```python
from build123d import *

# Parameters (mm, degrees)
F0_R     = 19.05
F0_R_2   = 6.35
F1_DEPTH = 134.62
F0_R_3   = 31.75
F2_DEPTH = 65.024
F3_R     = 5.08
F4_DEPTH = 114.3
F5_DEPTH = 89.662


with BuildPart() as f1:
    # F0 (on Front) → F1 (new body)
    with BuildSketch(Plane.XZ):
        Circle(F0_R)
        Circle(F0_R_2, mode=Mode.SUBTRACT)
    extrude(amount=F1_DEPTH)

    # F0 (on Front) → F2 (join)
    with BuildSketch(Plane.XZ):
        Circle(F0_R_3)
        Circle(F0_R, mode=Mode.SUBTRACT)
    extrude(amount=F2_DEPTH)

    # F3 (on Right) → F4 (cut)
    with BuildSketch(Plane.YZ):
        with Locations((-15.709256, 0)):
            Circle(F3_R)
        with Locations((-36.759584, 0)):
            Circle(F3_R)
    extrude(amount=-F4_DEPTH, mode=Mode.SUBTRACT)

    # F3 (on Right) → F5 (cut)
    with BuildSketch(Plane.YZ):
        with Locations((-15.709256, 0)):
            Circle(F3_R)
        with Locations((-36.759584, 0)):
            Circle(F3_R)
    extrude(amount=F5_DEPTH, mode=Mode.SUBTRACT)


solid = f1.part
```
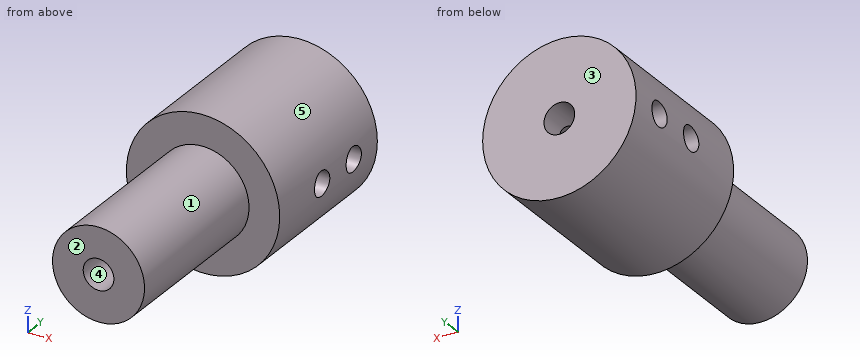
Can you work these out from the model? Positions are in its coordinate system, mm. Face numbers are marked on the shaded views. A direction names the side the tool comes from. Coordinates: 2 decimals unless noted, no trailing zeros. Order: outer loops, then holes, each group sorted by start corner. A loop starts at its lowest first (then second) coordinate and runs counter-clockwise, first axis right, second up. Notation, with made-up numbers: (-0.75, 35.25) -> (26.25, 35.25) arc R19 ccw to (26.25, 53.25) -> close; hole circle Ø5 at (56, -0.75). An arc over 180 degrees is marked (long way). Write each question's results on one line, items separated by ' | '.
Item 1: I want a section at B-B, the plane z = 0. Write out the boundary of the cut face in (x, y).
Results are:
outline: (-31.75, -65.02) -> (-19.05, -65.02) -> (-19.05, -134.62) -> (-6.35, -134.62) -> (-6.35, -41.84) -> (-31.75, -41.84) -> close; (-31.75, -31.68) -> (-6.35, -31.68) -> (-6.35, -20.79) -> (-31.75, -20.79) -> close; (-31.75, -10.63) -> (-6.35, -10.63) -> (-6.35, 0) -> (-31.75, 0) -> close; (6.35, -134.62) -> (19.05, -134.62) -> (19.05, -65.02) -> (31.75, -65.02) -> (31.75, -41.84) -> (6.35, -41.84) -> close; (6.35, -31.68) -> (31.75, -31.68) -> (31.75, -20.79) -> (6.35, -20.79) -> close; (6.35, -10.63) -> (31.75, -10.63) -> (31.75, 0) -> (6.35, 0) -> close
Item 2: I want a section at D-D, the plane x = 9.5. Write out the boundary of the cut face in (y, z).
Results are:
outline: (-134.62, -16.51) -> (-65.02, -16.51) -> (-65.02, -30.3) -> (0, -30.3) -> (0, 30.3) -> (-65.02, 30.3) -> (-65.02, 16.51) -> (-134.62, 16.51) -> close; hole circle Ø10.16 at (-36.76, 0); hole circle Ø10.16 at (-15.71, 0)
Item 3: I'm going to push flat-ended pins straight in: pin 1 Ø6 at (y, z) = (-91.5, 7) entering from -X; pin 2 Ø16.5 at (y, z) = (-15.71, 0) entering from +X; pin 3 Ø1 at (y, z) = (-98, -13.5) entering from +X; pin 4 Ø5 at (y, z) = (-63.5, -24) entering from +X. Where does each tip first touch, or does it pass through?
Results are:
pin 1: x = -18.63 | pin 2: x = 31.75 | pin 3: x = 13.92 | pin 4: x = 23.36
Item 4: I want a section at C-C, the plane y = -89. Write out the boundary of the cut face in (x, z), then the cut area to 3 significant figures.
Results are:
outline: circle Ø38.1 at (0, 0); hole circle Ø12.7 at (0, 0) | area: 1,010 mm²
Item 5: If we mould it in two halves opening along Z, with no side actions, what happens to the marked faces 3, 4 and 5? For each: +Z half, -Z half, draft (parallel to the pull), parting line (faces both ways), or undercut.
Results are:
face 3: draft | face 4: undercut | face 5: parting line
Item 6: If I drill on line 1 along Y through (x, z) = (20, 0); line 2 along Z through (x, y) = (0, -97); line 3 along Z through (x, y) = (0.5, -9), over which ranges is the centre line in solid material (lowest first)?
Results are:
line 1: -65.02 to -41.84, -31.68 to -20.79, -10.63 to 0 | line 2: -19.05 to -6.35, 6.35 to 19.05 | line 3: -31.75 to -6.33, 6.33 to 31.75
Item 7: I want a section at A-A, the plane x = 0. Write out the boundary of the cut face in (y, z).
Results are:
outline: (-134.62, -19.05) -> (-65.02, -19.05) -> (-65.02, -31.75) -> (0, -31.75) -> (0, -6.35) -> (-134.62, -6.35) -> close; (-134.62, 6.35) -> (0, 6.35) -> (0, 31.75) -> (-65.02, 31.75) -> (-65.02, 19.05) -> (-134.62, 19.05) -> close
Item 8: Which directions (+Z, -Z, +X, -X, +Y, -Y) give clear straight access to the entire face, cutting with the end or side of a thin tool? Please do the marked faces 1 and 2.
Results are:
face 1: -Y | face 2: +Z, -Z, +X, -X, -Y
